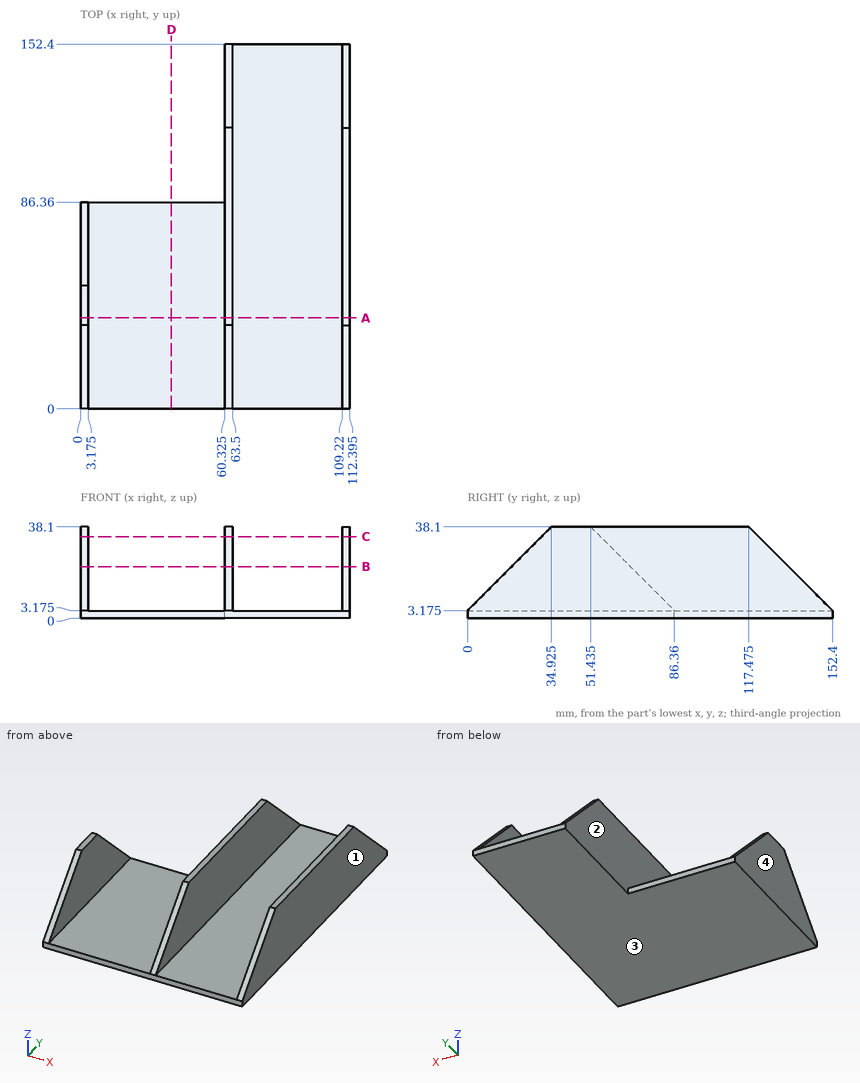
Drawing for the job (mm, zero at the part's lowest x, y, z). Give positions to 0.01 mm unless a question says otherwise; leave off trailing zeros. Loops run counter-clockwise (first coordinate to the right, second up) from the corner with the lowest first, then second, coordinate; pieces in that order, holes last.
Item 1: Slice it at A-A (y = 38). Write the cut outline in (x, z) (3 decimals), plus the area to 3 significant figures.
Check values:
outline: (0, 0) - (112.395, 0) - (112.395, 38.1) - (109.22, 38.1) - (109.22, 3.175) - (63.5, 3.175) - (63.5, 38.1) - (60.325, 38.1) - (60.325, 3.175) - (3.175, 3.175) - (3.175, 38.1) - (0, 38.1) - close
area: 690 mm2
Item 2: Mould opens along X. For the marked faces 1, 2, 3 and 4 say: +X half, -X half, draft (parallel to the pull), parting line (faces both ways), or undercut.
Check values:
face 1: +X half
face 2: undercut
face 3: draft
face 4: -X half
Item 3: Drill centre lines: line 1 along X through (y, z) = (14, 6) (3 decimals); line 2 along X through (y, z) = (109.5, 25) (3 decimals); line 3 along Z through (x, y) = (79, 108) (3 decimals). Where is each one in solid material? Low to high.
Check values:
line 1: x = 0 to 3.175, 60.325 to 63.5, 109.22 to 112.395
line 2: x = 60.325 to 63.5, 109.22 to 112.395
line 3: z = 0 to 3.175
Item 4: Slice it at B-B (z = 21.5). Write the cut outline in (x, y) (3 decimals).
Check values:
outline: (0, 18.325) - (3.175, 18.325) - (3.175, 68.035) - (0, 68.035) - close; (60.325, 18.325) - (63.5, 18.325) - (63.5, 134.075) - (60.325, 134.075) - close; (109.22, 18.325) - (112.395, 18.325) - (112.395, 134.075) - (109.22, 134.075) - close
Item 5: Slice it at C-C (z = 34). Write the cut outline in (x, y) (3 decimals).
Check values:
outline: (0, 30.825) - (3.175, 30.825) - (3.175, 55.535) - (0, 55.535) - close; (60.325, 30.825) - (63.5, 30.825) - (63.5, 121.575) - (60.325, 121.575) - close; (109.22, 30.825) - (112.395, 30.825) - (112.395, 121.575) - (109.22, 121.575) - close
Item 6: Drop flat-ended pins along their axis: P1, Ø4, axis at x = 42.5, y = 33.5, coming from the -Z side; P2, Ø1, axis at x = 21, z = 1.5, coming from the +Y side; P3, Ø17.5, axis at y = 101.5, z = 29, coming from the -X side (3 decimals); P4, Ø17, axis at x = 21, y = 38.5, coming from the +Z side (3 decimals). Give the stop position or say it passes through.
Check values:
P1: stops at z = 0
P2: stops at y = 86.36
P3: stops at x = 60.325
P4: stops at z = 3.175
Item 7: Slice it at D-D (x = 38). Write the cut outline in (y, z) (3 decimals).
Check values:
outline: (0, 0) - (86.36, 0) - (86.36, 3.175) - (0, 3.175) - close
